Geometry: see drawing. Coordinates: mm, zero at the bounding-box minimum. A direction names the side the tool comes from. Round coordinates to 2 decimals unless told otherwise and drop trailing zeros. Loops run counter-clockwise (first coordinate to the right, second up) from the corner with the lowest first, then second, coordinate; pieces in that order, holes last. Notation, with made-up numbers: (7.25, -28) -> (44.25, -28) arc R13 ccw to (44.25, -3) -> close; hole circle Ø7 at (81.5, 39). An arc over 180 degrees is marked (long way). Answer in a Markdown table with one row per item.
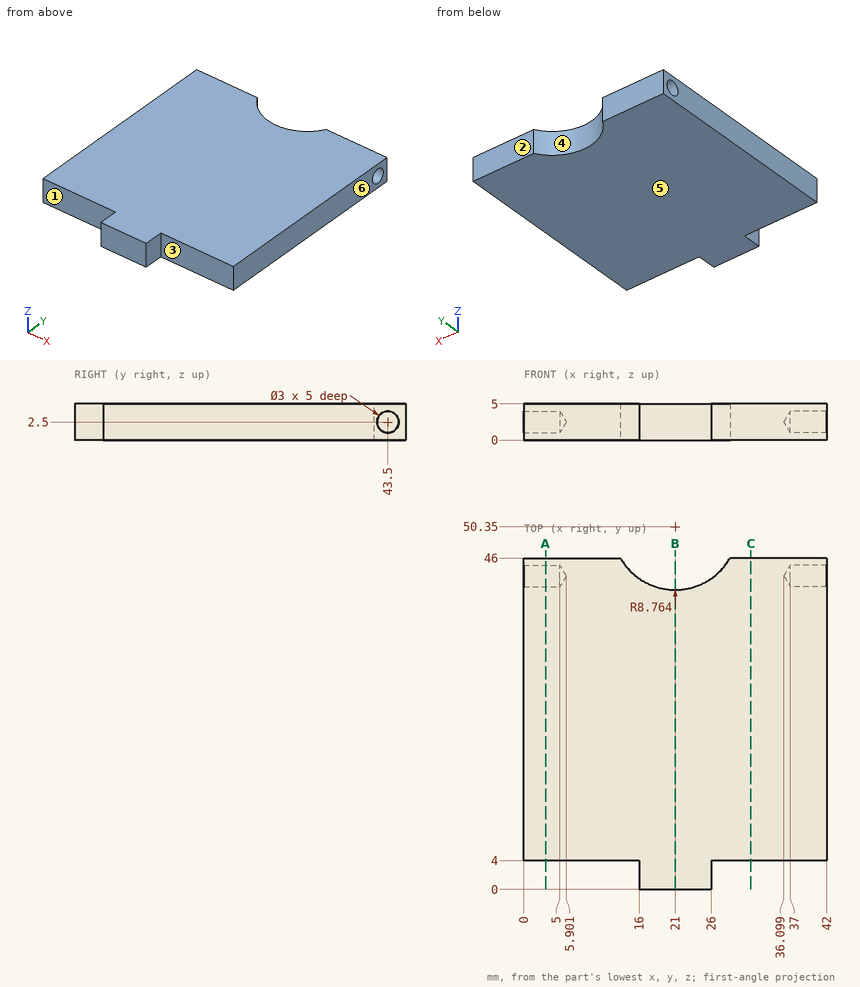
Item 1: Section query B-B, the plane x = 21. Output: boundary loops of the cut face in (y, z), and give its area (3 significant figures).
Ans:
| item | result |
|---|---|
| outline | (0, 0) -> (41.59, 0) -> (41.59, 5) -> (0, 5) -> close |
| area | 208 mm2 |
Item 2: Ray query, L1, parallel to Y at x = 1.5, z = 2.5; L2, parallel to Z at x = 1.2, y = 43.5; L3, parallel to Y at x = 12, z = 0.25. Return the intervals inside material, ascending.
Ans:
| item | result |
|---|---|
| L1 | 4 to 42, 45 to 46 |
| L2 | 0 to 1, 4 to 5 |
| L3 | 4 to 46 |
Item 3: Section query C-C, the plane x = 31.5. Output: boundary loops of the cut face in (y, z).
Ans:
| item | result |
|---|---|
| outline | (4, 0) -> (46, 0) -> (46, 5) -> (4, 5) -> close |
Item 4: Mould query, pull axis X, two halves, no side actions, for the marked faces 4, 5 and 6. Classes: released by +X, released by -X, zero draft, split by the parting line, or undercut.
Ans:
| item | result |
|---|---|
| face 4 | undercut |
| face 5 | zero draft |
| face 6 | released by +X |
Item 5: Section query A-A, the plane x = 3. Output: boundary loops of the cut face in (y, z), and give its area (3 significant figures).
Ans:
| item | result |
|---|---|
| outline | (4, 0) -> (46, 0) -> (46, 5) -> (4, 5) -> close; hole circle Ø3 at (43.5, 2.5) |
| area | 203 mm2 |
Item 6: First-contact query: P1, Ø3, axis at y = 1, z = 2, coming from the -X side; P2, Ø8, axis at x = 33, y = 20.5, coming from the -Z side; P3, Ø1.5, axis at x = 9.5, z = 2, coming from the -Y side; P4, Ø1.2, axis at y = 1, z = 3.5, coming from the +X side. Flat tips, straight axial feed; report the tip coordinate or a pass-through.
Ans:
| item | result |
|---|---|
| P1 | x = 16 |
| P2 | z = 0 |
| P3 | y = 4 |
| P4 | x = 26 |
Item 7: Set-up query: the marked faces 1, 2 and 3. Return all of +Z, -Z, +X, -X, +Y, -Y with unobstructed straight access to the full face (end or side cutting, diameter ignored); none if empty.
Ans:
| item | result |
|---|---|
| face 1 | +Z, -Z, -X, -Y |
| face 2 | +Z, -Z, +X, -X, +Y |
| face 3 | +Z, -Z, +X, -Y |
